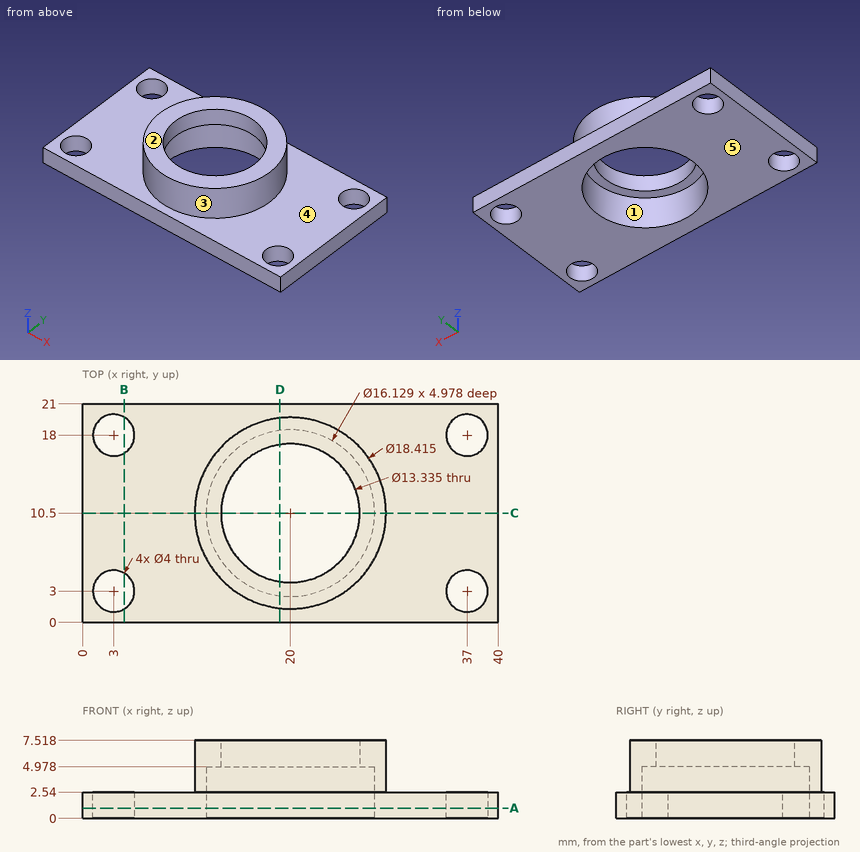
The drawing under review shows one solid part. Ordinate dimensions are in mm from its lowest x, y, z. A direction names the side the tool comes from. Give positions to 0.01 mm unless a question says otherwise; leave off trailing zeros. Loops run counter-clockwise (first coordinate to the right, second up) from the corner with the lowest first, then second, coordinate; pieces in that order, holes last. Notation, with made-up numbers: M 30,7.25 L 66,7.25 A24 cw 66,31.25 Z; hole C 27,-30.75 d8. An arc over 180 degrees is marked long. Return JSON: item names as keys, results as strings. Group by question number.
Item 1: We need section B-B (x = 4). Give the boundary of the cut face in (y, z).
Item 2: Insertion check: pin 1 Ø1.5 at (x, z) = (20, 6) entering from -Y; pin 2 Ø3.5 at (x, y) = (37, 3) entering from -Z; pin 3 Ø2 at (y, z) = (18.5, 4) entering from +X; pin 4 Ø2 at (y, z) = (17, 5) entering from +X (1 decimal). Each pin has a flat end and moves straight along its axis. Give the tip position at first contact, or say it passes through.
Item 3: We need section C-C (y = 10.5). Give the boundary of the cut face in (x, z) (1 decimal).
Item 4: We need section A-A (z = 1). Give the boundary of the cut face in (x, y) (1 decimal).
Item 5: Tool access review of the marked faces 4 and 5: name each direction out of +Z, -Z, +X, -X, +Y, -Y from which nothing blocks a thin tool from reaching the whole face with its end or side.
Item 6: For probe 1 along X at (y, z) = (10.5, 1) (1 decimal); probe 2 along X at (y, z) = (19, 2); probe 3 along X at (y, z) = (16, 3.25) (1 decimal), list the stretches that pass through material, from the lowest coordinate up.
Item 7: We need section D-D (x = 19). Give the boundary of the cut face in (y, z), and give its area (3 significant figures).
Item 8: Mouldability with a two-part tool opening along X and no side actions: class the marked faces 1, 2 and 3 as released by +X, released by -X, zero draft, split by the parting line, or undercut.
Output:
{
 "1": {"outline": "M 0,0 L 1.27,0 L 1.27,2.54 L 0,2.54 Z; M 4.73,0 L 16.27,0 L 16.27,2.54 L 4.73,2.54 Z; M 19.73,0 L 21,0 L 21,2.54 L 19.73,2.54 Z"},
 "2": {"pin 1": "stops at y = 1.29", "pin 2": "passes through", "pin 3": "stops at x = 25.98", "pin 4": "stops at x = 27.4"},
 "3": {"outline": "M 0,0 L 11.9,0 L 11.9,5 L 13.3,5 L 13.3,7.5 L 10.8,7.5 L 10.8,2.5 L 0,2.5 Z; M 26.7,5 L 28.1,5 L 28.1,0 L 40,0 L 40,2.5 L 29.2,2.5 L 29.2,7.5 L 26.7,7.5 Z"},
 "4": {"outline": "M 0,0 L 40,0 L 40,21 L 0,21 Z; hole C 3,3 d4; hole C 3,18 d4; hole C 20,10.5 d16.1; hole C 37,3 d4; hole C 37,18 d4"},
 "5": {"face 4": "+Z", "face 5": "-Z, +X, -X, +Y, -Y"},
 "6": {"probe 1": "x = 0 to 11.9, 28.1 to 40", "probe 2": "x = 0 to 1.27, 4.73 to 35.27, 38.73 to 40", "probe 3": "x = 12.6 to 14.1, 25.9 to 27.4"},
 "7": {"outline": "M 0,0 L 2.5,0 L 2.5,4.98 L 3.91,4.98 L 3.91,7.52 L 1.35,7.52 L 1.35,2.54 L 0,2.54 Z; M 17.09,4.98 L 18.5,4.98 L 18.5,0 L 21,0 L 21,2.54 L 19.65,2.54 L 19.65,7.52 L 17.09,7.52 Z", "area": "31.3 mm^2"},
 "8": {"face 1": "undercut", "face 2": "zero draft", "face 3": "split by the parting line"}
}
